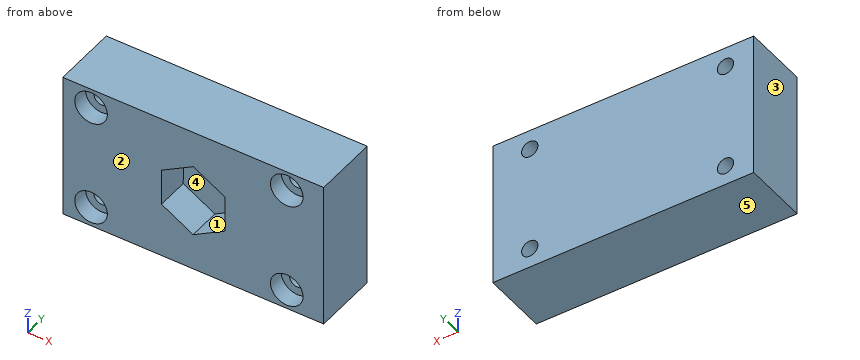
```python
from build123d import *

# Parameters (mm, degrees)
F0_W           = 101.6
F0_H           = 57.15
F1_DEPTH       = 25.4
F3_D           = 6.35
F3_CBORE_D     = 12.7
F3_CBORE_DEPTH = 6.35
F5_DEPTH       = 12.7


with BuildPart() as f1:
    # F0 (on Front) → F1 (new body)
    with BuildSketch(Plane.XZ):
        Rectangle(F0_W, F0_H)
    extrude(amount=F1_DEPTH)

    # F3 (through all)
    with Locations(Plane.XZ.offset(25.4)):
        with Locations((36.4028997615, 20.831474103), (36.4028997615, -20.831474103), (-39.7971002385, 20.831474103), (-39.7971002385, -20.831474103)):
            CounterBoreHole(F3_D / 2, F3_CBORE_D / 2, F3_CBORE_DEPTH)

    # F4 (on face) → F5 (cut)
    with BuildSketch(Plane.XZ.offset(25.4)):
        Polygon((-0.0431249981, -14.2548758505), (12.3235221152, -7.1647852691), (12.3666471133, 7.0900905813), (0.0431249981, 14.2548758505), (-12.3235221152, 7.1647852691), (-12.3666471133, -7.0900905813), align=None)
    extrude(amount=-F5_DEPTH, mode=Mode.SUBTRACT)


solid = f1.part
```
Can you work these out from the model? Positions are in its coordinate system, mm. Face numbers are marked on the shaded views. A direction names the side the tool comes from. Round coordinates to 2 decimals unless told otherwise and drop trailing zeros. Loops run counter-clockwise (first coordinate to the right, second up) from the corner with the lowest first, then second, coordinate; pieces in that order, holes last. Notation, with made-up numbers: M 35,-30 L 63,-30 A23 cw 63,7 Z; hole C 31,82 d4. An arc over 180 degrees is marked long. Answer as a JSON object with one key per item and string values. Group by question number.
Q1. Please list where these lines run through material, in increasing order: L1, parallel to X at y = -21, z = -21; L2, parallel to X at y = -8.5, z = -23; L3, parallel to X at y = -15.5, z = -1.
Q2. Imagine slicing it at C-C, the plane y = -16.25. Please give me the cut outline in (x, z) (3 decimals), then the cut area to 3 significant figures.
Q3. On a 3-axis mill with a long thin cutter (end or side, diameter ignored), from which of +Z, -Z, +X, -X, +Y, -Y can I reach the whole of each face in a straight line? I mean the marked faces 1 and 2. Say none if no direction works.
Q4. We'd pull the mould along Z, two halves only. Please class the marked faces 3, 4 and 5: +Z half, -Z half, draft (parallel to the pull), parting line (faces both ways), or undercut.
Q5. Imagine slicing it at B-B, the plane x = -39.5. Please give me the cut outline in (y, z) (3 decimals).
Q6. Will these pins go through, and if not, where does the flat tip stop? pin 1 (7.5 mm diameter, centred on x = 3, z = 2.5, fed in from -Y); pin 2 (4 mm diameter, centred on x = 34.5, z = 18.5, fed in from -Y).
Q7. Imagine slicing it at A-A, the plane z = 22.5. Please give me the cut outline in (x, y), then the cut area to 3 significant figures.
Q8. Imagine slicing it at D-D, the plane y = -10.25. Please give me the cut outline in (x, z) (3 decimals), then the cut area to 3 significant figures.
Findings:
{
 "1": {"L1": "x = -50.8 to -46.14, -33.45 to 30.06, 42.75 to 50.8", "L2": "x = -50.8 to -42.12, -37.48 to 34.08, 38.72 to 50.8", "L3": "x = -50.8 to -12.35, 12.34 to 50.8"},
 "2": {"outline": "M -50.8,-28.575 L 50.8,-28.575 L 50.8,28.575 L -50.8,28.575 Z; hole C -39.797,-20.831 d6.35; hole C -39.797,20.831 d6.35; hole M -12.367,-7.09 L -0.043,-14.255 L 12.324,-7.165 L 12.367,7.09 L 0.043,14.255 L -12.324,7.165 Z; hole C 36.403,-20.831 d6.35; hole C 36.403,20.831 d6.35", "area": "5,150 mm2"},
 "3": {"face 1": "-Y", "face 2": "+Z, -Z, +X, -X, -Y"},
 "4": {"face 3": "draft", "face 4": "undercut", "face 5": "-Z half"},
 "5": {"outline": "M -25.4,-28.575 L 0,-28.575 L 0,-23.993 L -19.05,-23.993 L -19.05,-27.175 L -25.4,-27.175 Z; M -25.4,-14.488 L -19.05,-14.488 L -19.05,-17.67 L 0,-17.67 L 0,17.67 L -19.05,17.67 L -19.05,14.488 L -25.4,14.488 Z; M -25.4,27.175 L -19.05,27.175 L -19.05,23.993 L 0,23.993 L 0,28.575 L -25.4,28.575 Z"},
 "6": {"pin 1": "stops at y = -12.7", "pin 2": "stops at y = -19.05"},
 "7": {"outline": "M -50.8,-25.4 L -45.92,-25.4 L -45.92,-19.05 L -42.5,-19.05 L -42.5,0 L -50.8,0 Z; M -37.1,-19.05 L -33.67,-19.05 L -33.67,-25.4 L 30.28,-25.4 L 30.28,-19.05 L 33.7,-19.05 L 33.7,0 L -37.1,0 Z; M 39.1,-19.05 L 42.53,-19.05 L 42.53,-25.4 L 50.8,-25.4 L 50.8,0 L 39.1,0 Z", "area": "2,220 mm2"},
 "8": {"outline": "M -50.8,-28.575 L 50.8,-28.575 L 50.8,28.575 L -50.8,28.575 Z; hole C -39.797,-20.831 d6.35; hole C -39.797,20.831 d6.35; hole C 36.403,-20.831 d6.35; hole C 36.403,20.831 d6.35", "area": "5,680 mm2"}
}
